```python
from build123d import *

# Parameters (mm, degrees)
F0_W     = 50.8
F0_H     = 38.1
F1_DEPTH = 31.75
F3_DEPTH = 12.7
F5_DEPTH = 25.4
F6_DEPTH = 6.35


with BuildPart() as f1:
    # F0 (on Front) → F1 (new body)
    with BuildSketch(Plane.XZ):
        with Locations((-45.7247960726, 26.2155969156)):
            Rectangle(F0_W, F0_H)
    extrude(amount=F1_DEPTH)

    # F2 (on face) → F3 (cut)
    with BuildSketch(Plane.XZ.offset(31.75)):
        Polygon((-45.7247960726, 45.2655969156), (-20.3247960726, 7.1655969156), (-20.3247960726, 45.2655969156), align=None)
    extrude(amount=-F3_DEPTH, mode=Mode.SUBTRACT)

    # F4 (on face) → F5 (cut)
    with BuildSketch(Plane.XZ.offset(19.05)):
        Polygon((-45.7247960726, 45.2655969156), (-33.0247960726, 26.2155969156), (-20.3247960726, 26.2155969156), (-20.3247960726, 45.2655969156), align=None)
    extrude(amount=-F5_DEPTH, mode=Mode.SUBTRACT)

    # F6 (add): a face of the model
    f6_faces = [f1.faces().sort_by_distance(p)[0] for p in [
        (-20.3247960726, -9.525, 16.6905969156),
    ]]
    extrude(f6_faces, amount=F6_DEPTH)


solid = f1.part
```
Geometry check sheet. Reference: the model listing, model coordinates, mm. A direction names the side the tool comes from. Coordinates: 2 decimals unless noted, no trailing zeros. Order: outer loops, then holes, each group sorted by start corner. A loop starts at its lowest first (then second) coordinate and runs counter-clockwise, first axis right, second up. Notation, with made-up numbers: (-33, 42) - (-8, 42) arc R21 cw to (-8, 66) - close; hole circle Ø4 at (40.25, 37). An arc over 180 degrees is marked (long way). Use one line per item in the form item = value.
1. Access from +Z, -Z, +X, -X, +Y, -Y to the whole of each face (thin tool, end or side, straight path). Record for faces 1 (the face through (-22, -19.05, 19)), 2 (the face through (-24, -10, 26.216)), 3 (the face through (-49, 0, 22)).
Here are the results:
face_1 = +Z, +X, -Y
face_2 = +Z, +X, +Y, -Y
face_3 = +Z, -Z, +X, -X, +Y
2. Section check D-D (y = -21). Record the boundary of the cut face in (x, z), then the cut area to 3 significant figures.
Here are the results:
outline = (-71.12, 7.17) - (-20.32, 7.17) - (-45.72, 45.27) - (-71.12, 45.27) - close
area = 1,450 mm²
3. Section check B-B (z = 21.5). Record the boundary of the cut face in (x, y), then the cut area to 3 significant figures.
Here are the results:
outline = (-71.12, -31.75) - (-29.88, -31.75) - (-29.88, -19.05) - (-13.97, -19.05) - (-13.97, 0) - (-71.12, 0) - close
area = 1,610 mm²
4. Section check A-A (y = -14.5). Record the boundary of the cut face in (x, z).
Here are the results:
outline = (-71.12, 7.17) - (-13.97, 7.17) - (-13.97, 26.22) - (-33.02, 26.22) - (-45.72, 45.27) - (-71.12, 45.27) - close
5. Gauge pin test, flat ends, axial feed: pin 1 (9.5 mm diameter, centred on x = -23.5, z = 14.5, fed in from -Y); pin 2 (6 mm diameter, centred on y = -25.5, z = 17.5, fed in from +X); pin 3 (2 mm diameter, centred on y = -6, z = 41, fed in from +X); pin 4 (5 mm diameter, centred on x = -28.5, y = -12.5, fed in from +Z). Record the tip position at first contact, or that the pin passes through.
Here are the results:
pin_1 = -31.75
pin_2 = -25.21
pin_3 = -42.21
pin_4 = 26.22
6. Section check C-C (x = -38.5). Record the boundary of the cut face in (y, z), then the cut area to 3 significant figures.
Here are the results:
outline = (-31.75, 7.17) - (0, 7.17) - (0, 34.43) - (-31.75, 34.43) - close
area = 866 mm²
7. Scan lines: line 1 (Z direction, x = -21.5, y = -9.5); line 2 (Y direction, x = -18.5, z = 22); line 3 (X direction, y = -9, z = 42). Record each from-to range of solid material in increasing order.
Here are the results:
line_1 = 7.17 to 26.22
line_2 = -19.05 to 0
line_3 = -71.12 to -43.55
